```python
from build123d import *

# Parameters (mm, degrees)
F0_R     = 10
F1_DEPTH = 1
F3_DEPTH = 0.7
F4_DEPTH = 1


with BuildPart() as f1:
    # F0 (on Front) → F1 (new body)
    with BuildSketch(Plane.XZ):
        Circle(F0_R)
    extrude(amount=F1_DEPTH)

    # F2 (on Front) → F3 (cut)
    with BuildSketch(Plane.XZ):
        Polygon((2.3, 5.581941), (0, 5.581941), (-2.3, 5.581941), (-3.99405, 3.847297), (-3.858357, -3.854667), (-2.3, -5.414516), (2.289638, -5.414516), (3.85098, -3.854667), (3.85098, 3.847297), align=None)
    extrude(amount=-F3_DEPTH, mode=Mode.SUBTRACT)

    # F2 (on Front) → F4 (cut)
    with BuildSketch(Plane.XZ):
        Polygon((2.3, 5.581941), (0, 5.581941), (-2.3, 5.581941), (-3.99405, 3.847297), (-3.858357, -3.854667), (-2.3, -5.414516), (2.289638, -5.414516), (3.85098, -3.854667), (3.85098, 3.847297), align=None)
    extrude(amount=F4_DEPTH, mode=Mode.SUBTRACT)


solid = f1.part
```
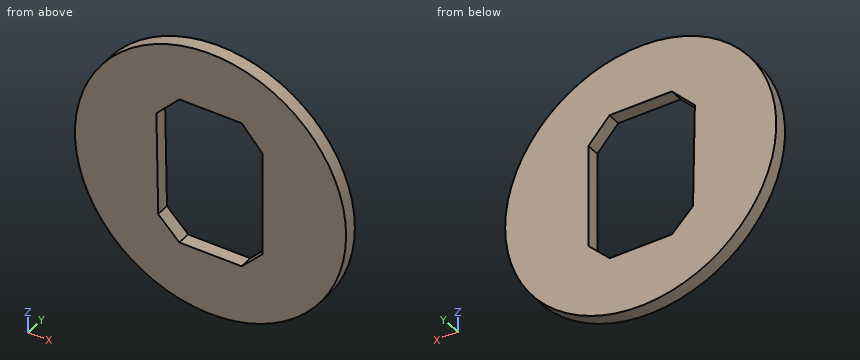
The listing builds one solid part. Answer for the finished solid, in the listing's coordinates (mm). Round coordinates to 2 decimals unless told otherwise and drop trailing zeros. Loops run counter-clockwise (first coordinate to the right, second up) from the corner with the lowest first, then second, coordinate; pieces in that order, holes last. Notation, with made-up numbers: (84, 30) - (111, 30) arc R17 cw to (111, 62) - close; hole circle Ø1 at (28, -29). An arc over 180 degrees is marked (long way). Use one line per item in the form item = value. Start each with the question number.
1. The part is cut by section D-D on x = 6. Determine the outline of the cut face in (y, z).
2. The part is cut by section B-B on x = 0. Determine the outline of the cut face in (y, z).
3. The part is cut by section C-C on z = 0. Determine the outline of the cut face in (x, y), then the cut area to 3 significant figures.
4. The part is cut by section A-A on y = -0.8. Determine the outline of the cut face in (x, z), then the cut area to 3 significant figures.
5. Consider line 1 (Z direction, x = -0.25, y = -0.4); line 2 (X direction, y = -0.1, z = 5.5); line 3 (Z direction, x = -1.25, y = -0.4). Determine where each line is inside the solid, lowest interval first. Write a range as [from, to].
Geometry check:
q1.outline = (-1, -8) - (0, -8) - (0, 8) - (-1, 8) - close
q2.outline = (-1, -10) - (0, -10) - (0, -5.41) - (-1, -5.41) - close; (-1, 5.58) - (0, 5.58) - (0, 10) - (-1, 10) - close
q3.outline = (-10, -1) - (-3.93, -1) - (-3.93, 0) - (-10, 0) - close; (3.85, -1) - (10, -1) - (10, 0) - (3.85, 0) - close
q3.area = 12.2 mm^2
q4.outline = circle Ø20 at (0, 0); hole (-3.99, 3.85) - (-3.86, -3.85) - (-2.3, -5.41) - (2.29, -5.41) - (3.85, -3.85) - (3.85, 3.85) - (2.3, 5.58) - (-2.3, 5.58) - close
q4.area = 234 mm^2
q5.line_1 = [-10, -5.41], [5.58, 10]
q5.line_2 = [-8.35, -2.38], [2.37, 8.35]
q5.line_3 = [-9.92, -5.41], [5.58, 9.92]
